Verification items for the finished model (mm, model axes). A direction names the side the tool comes from. Give positions to 0.01 mm unless a question says otherwise; leave off trailing zeros. Loops run counter-clockwise (first coordinate to the right, second up) from the corner with the lowest first, then second, coordinate; pieces in that order, holes last. Notation, with made-up numbers: (22, -6.5) - (61, -6.5) arc R13 ccw to (61, 2.5) - close; hole circle Ø1 at (80.25, -26.5). An arc over 180 degrees is marked (long way). Use one line per item in the form item = value.
```python
from build123d import *

# Parameters (mm, degrees)
BODY_DEPTH        = 17.3
BODY_2_DEPTH      = 17.3
SKETCH2_W         = 7.5
SKETCH2_H         = 5
END_DEPTH         = 1.2
END1_START        = 17.3
SKETCH2_4_W       = 7.5
SKETCH2_4_H       = 5
END1_DEPTH        = 1.2
SKETCH3_R         = 0.75
TENDON_HOLE_DEPTH = 19.7


with BuildPart() as part:
    # Sketch1 → body (new body)
    with BuildSketch(Plane.XY):
        Polygon((3.75, 0), (3.75, 5), (2.25, 5), (2.25, 1.5), (0.6, 1.5), (0.6, 0), align=None)
    extrude(amount=BODY_DEPTH)



with BuildPart() as body_2_2:
    # Sketch1 → body 2 (new body)
    with BuildSketch(Plane.XY):
        Polygon((-2.25, 1.5), (-2.25, 5), (-3.75, 5), (-3.75, 0), (-0.6, 0), (-0.6, 1.5), align=None)
    extrude(amount=BODY_2_DEPTH)


with BuildPart() as part_1:
    add(part.part)

    add(body_2_2.part)  # end merges body 2 2
    # Sketch2 → end (add)
    with BuildSketch(Plane.XY):
        with Locations((0, 2.5)):
            Rectangle(SKETCH2_W, SKETCH2_H)
    extrude(amount=-END_DEPTH)

    # Sketch2<4> → end1 (add)
    with BuildSketch(Plane.XY.offset(END1_START)):
        with Locations((0, 2.5)):
            Rectangle(SKETCH2_4_W, SKETCH2_4_H)
    extrude(amount=END1_DEPTH)

    # Sketch3 → tendon hole (cut)
    with BuildSketch(Plane.XY.offset(18.5)):
        with Locations((0, 3.5)):
            Circle(SKETCH3_R)
    extrude(amount=-TENDON_HOLE_DEPTH, mode=Mode.SUBTRACT)


solid = part_1.part
```
1. Section check D-D, the plane y = 3.5. Record the cut outline in (x, z).
Result set:
outline = (-3.75, -1.2) - (-0.75, -1.2) - (-0.75, 0) - (-2.25, 0) - (-2.25, 17.3) - (-0.75, 17.3) - (-0.75, 18.5) - (-3.75, 18.5) - close; (0.75, -1.2) - (3.75, -1.2) - (3.75, 18.5) - (0.75, 18.5) - (0.75, 17.3) - (2.25, 17.3) - (2.25, 0) - (0.75, 0) - close
2. Tool access check on faces 1 (the flat face through (-0.6, 1, 9)), 2 (the flat face through (-2.25, 3, 9)), 3 (the cylindrical face through (-0.163, 2.768, 17.908)). Record the directions out of +Z, -Z, +X, -X, +Y, -Y that give a thin tool (end or side, any length) a straight path to the whole face; none if there is none.
Result set:
face_1 = +Y, -Y
face_2 = +Y
face_3 = +Z, -Z
3. Depth check by flat-ended pin: pin 1 Ø2 at (x, y) = (0, 3.5) entering from +Z; pin 2 Ø1.4 at (x, y) = (0, 3.5) entering from -Z; pin 3 Ø0.5 at (x, z) = (1, 7.5) entering from +Y. Enter the tip coordinate at first touch or a pass-through.
Result set:
pin_1 = 18.5
pin_2 = through
pin_3 = 1.5
4. Scan lines: probe 1 along Y at (x, z) = (0, -0.8); probe 2 along X at (y, z) = (3, 5); probe 3 along X at (y, z) = (0.7, 8.25). Record each from-to range of solid material in increasing order.
Result set:
probe_1 = 0 to 2.75, 4.25 to 5
probe_2 = -3.75 to -2.25, 2.25 to 3.75
probe_3 = -3.75 to -0.6, 0.6 to 3.75
5. Section check B-B, the plane y = 1.15. Record the cut outline in (x, z), then the cut area to 3 significant figures.
Result set:
outline = (-3.75, -1.2) - (3.75, -1.2) - (3.75, 18.5) - (-3.75, 18.5) - close; hole (-0.6, 0) - (0.6, 0) - (0.6, 17.3) - (-0.6, 17.3) - close
area = 127 mm²
6. Section check C-C, the plane z = 13.75. Record the cut outline in (x, y).
Result set:
outline = (-3.75, 0) - (-0.6, 0) - (-0.6, 1.5) - (-2.25, 1.5) - (-2.25, 5) - (-3.75, 5) - close; (0.6, 0) - (3.75, 0) - (3.75, 5) - (2.25, 5) - (2.25, 1.5) - (0.6, 1.5) - close
7. Draft check along X on faces 4 (the flat face through (3.75, 2, 9)), 5 (the flat face through (1, 1.5, 9)), 6 (the cylindrical face through (-0.163, 2.768, -0.592)), 7 (the flat face through (-0.1, 2.5, 18.5)). Enter one of: released by +X, released by -X, zero draft, split by the parting line, or undercut.
Result set:
face_4 = released by +X
face_5 = undercut
face_6 = undercut
face_7 = zero draft
8. Section check A-A, the plane x = 0. Record the cut outline in (y, z).
Result set:
outline = (0, -1.2) - (2.75, -1.2) - (2.75, 0) - (0, 0) - close; (0, 17.3) - (2.75, 17.3) - (2.75, 18.5) - (0, 18.5) - close; (4.25, -1.2) - (5, -1.2) - (5, 0) - (4.25, 0) - close; (4.25, 17.3) - (5, 17.3) - (5, 18.5) - (4.25, 18.5) - close
